```python
from build123d import *

# Parameters (mm, degrees)
BOSS_EXTRUDE3_DEPTH = 7.8
SKETCH2_R           = 2.4
CUT_EXTRUDE4_DEPTH  = 7.8
SKETCH3_R           = 3.05
CUT_EXTRUDE5_DEPTH  = 0.8
SKETCH4_R           = 3.05
CUT_EXTRUDE6_DEPTH  = 0.8


with BuildPart() as part:
    # Sketch1 → Boss-Extrude3 (new body)
    with BuildSketch(Plane(origin=(0, 0, 0), x_dir=(1, 0, 0), z_dir=(0, 1, 0))):
        with BuildLine():
            Line((-16, -3.7), (80, -3.7))
            ThreePointArc((80, -3.7), (83.7, 0), (80, 3.7))
            Line((80, 3.7), (-16, 3.7))
            ThreePointArc((-16, 3.7), (-19.7, 0), (-16, -3.7))
        make_face()
    extrude(amount=BOSS_EXTRUDE3_DEPTH)

    # Sketch2 → Cut-Extrude4 (cut)
    with BuildSketch(Plane(origin=(0, 7.8, 0), x_dir=(1, 0, 0), z_dir=(0, 1, 0))):
        Circle(SKETCH2_R)
        with Locations((8, 0)):
            Circle(SKETCH2_R)
        with Locations((16, 0)):
            Circle(SKETCH2_R)
        with Locations((-16, 0)):
            Circle(SKETCH2_R)
        with Locations((-8, 0)):
            Circle(SKETCH2_R)
        with Locations((24, 0)):
            Circle(SKETCH2_R)
        with Locations((32, 0)):
            Circle(SKETCH2_R)
        with Locations((40, 0)):
            Circle(SKETCH2_R)
        with Locations((48, 0)):
            Circle(SKETCH2_R)
        with Locations((56, 0)):
            Circle(SKETCH2_R)
        with Locations((64, 0)):
            Circle(SKETCH2_R)
        with Locations((72, 0)):
            Circle(SKETCH2_R)
        with Locations((80, 0)):
            Circle(SKETCH2_R)
    extrude(amount=-CUT_EXTRUDE4_DEPTH, mode=Mode.SUBTRACT)

    # Sketch3 → Cut-Extrude5 (cut)
    with BuildSketch(Plane(origin=(0, 7.8, 0), x_dir=(1, 0, 0), z_dir=(0, 1, 0))):
        Circle(SKETCH3_R)
        with Locations((8, 0)):
            Circle(SKETCH3_R)
        with Locations((16, 0)):
            Circle(SKETCH3_R)
        with Locations((-16, 0)):
            Circle(SKETCH3_R)
        with Locations((-8, 0)):
            Circle(SKETCH3_R)
        with Locations((32, 0)):
            Circle(SKETCH3_R)
        with Locations((24, 0)):
            Circle(SKETCH3_R)
        with Locations((40, 0)):
            Circle(SKETCH3_R)
        with Locations((48, 0)):
            Circle(SKETCH3_R)
        with Locations((56, 0)):
            Circle(SKETCH3_R)
        with Locations((64, 0)):
            Circle(SKETCH3_R)
        with Locations((72, 0)):
            Circle(SKETCH3_R)
        with Locations((80, 0)):
            Circle(SKETCH3_R)
    extrude(amount=-CUT_EXTRUDE5_DEPTH, mode=Mode.SUBTRACT)

    # Sketch4 → Cut-Extrude6 (cut)
    with BuildSketch(Plane.XZ):
        Circle(SKETCH4_R)
        with Locations((8, 0)):
            Circle(SKETCH4_R)
        with Locations((16, 0)):
            Circle(SKETCH4_R)
        with Locations((-16, 0)):
            Circle(SKETCH4_R)
        with Locations((-8, 0)):
            Circle(SKETCH4_R)
        with Locations((32, 0)):
            Circle(SKETCH4_R)
        with Locations((24, 0)):
            Circle(SKETCH4_R)
        with Locations((40, 0)):
            Circle(SKETCH4_R)
        with Locations((48, 0)):
            Circle(SKETCH4_R)
        with Locations((56, 0)):
            Circle(SKETCH4_R)
        with Locations((64, 0)):
            Circle(SKETCH4_R)
        with Locations((72, 0)):
            Circle(SKETCH4_R)
        with Locations((80, 0)):
            Circle(SKETCH4_R)
    extrude(amount=-CUT_EXTRUDE6_DEPTH, mode=Mode.SUBTRACT)


solid = part.part
```
Verification items for the finished model (mm, model axes). A direction names the side the tool comes from. Give positions to 0.01 mm unless a question says otherwise; leave off trailing zeros. Loops run counter-clockwise (first coordinate to the right, second up) from the corner with the lowest first, then second, coordinate; pieces in that order, holes last.
1. Section check B-B, the plane y = 2. Count the separate pieces of the cut face and the enclosed holes in it, then the cut area to 3 significant figures.
2. Section check D-D, the plane x = 49.5. Enter the section's corners in (y, z).
3. Thickness scan on line 1 (Z direction, x = 72, y = 7.3); line 2 (Z direction, x = 56, y = 5.5); line 3 (Y direction, x = -1, z = 2.25). Record the ranges inside material, lowest first.
4. Go/stop test with flat-tipped pins: pin 1 Ø1 at (y, z) = (2.5, 1.5) entering from +X; pin 2 Ø3 at (y, z) = (1, 1.5) entering from -X; pin 3 Ø3 at (x, z) = (57, 1) entering from -Y. Record where each tip stops, or that it passes through.
5. Set-up check for faces 4 (the flat face through (70, 7, 2)), 5 (the cylindrical face through (76.953, 0.394, 0.134)), 6 (the cylindrical face through (37.602, 3.943, -0.106)): record each of +Z, -Z, +X, -X, +Y, -Y from which the full face is reachable in a straight line by a thin tool's end or side.
6. Mould release check, pull along X, two halves, no side actions. Record for faces 1 (the cylindrical face through (-11.047, 7.406, -0.134)), 2 (the cylindrical face through (-19.7, 3.8, -0.1)), 3 (the cylindrical face through (26.29, 3.94, -0.72)): released by +X, released by -X, zero draft, split by the parting line, or undercut.
7. Section check A-A, the plane x = 32. Enter the section's corners in (y, z), then the cut area to 3 significant figures.
Geometry says:
1. separate pieces: 1
1. enclosed holes: 13
1. area: 518 mm2
2. outline: (0, -3.7) - (7.8, -3.7) - (7.8, -2.66) - (7, -2.66) - (7, -1.87) - (0.8, -1.87) - (0.8, -2.66) - (0, -2.66) - close; (0, 2.66) - (0.8, 2.66) - (0.8, 1.87) - (7, 1.87) - (7, 2.66) - (7.8, 2.66) - (7.8, 3.7) - (0, 3.7) - close
3. line 1: z = -3.7 to -3.05, 3.05 to 3.7
3. line 2: z = -3.7 to -2.4, 2.4 to 3.7
3. line 3: y = 0.8 to 7
4. pin 1: stops at x = 83.56
4. pin 2: stops at x = -19.7
4. pin 3: stops at y = 0.8
5. face 4: +Y
5. face 5: -Y
5. face 6: +Y, -Y
6. face 1: undercut
6. face 2: released by -X
6. face 3: undercut
7. outline: (0, -3.7) - (7.8, -3.7) - (7.8, -3.05) - (7, -3.05) - (7, -2.4) - (0.8, -2.4) - (0.8, -3.05) - (0, -3.05) - close; (0, 3.05) - (0.8, 3.05) - (0.8, 2.4) - (7, 2.4) - (7, 3.05) - (7.8, 3.05) - (7.8, 3.7) - (0, 3.7) - close
7. area: 18.2 mm2
